The listing builds one solid part. Answer for the finished solid, in the listing's coordinates (mm). A direction names the side the tool comes from. Give positions to 0.01 mm unless a question says otherwise; leave off trailing zeros. Order: outer loops, then holes, each group sorted by start corner. A loop starts at its lowest first (then second) coordinate and runs counter-clockwise, first axis right, second up.
```python
from build123d import *

# Parameters (mm, degrees)
F0_W         = 42
F0_H         = 54
F1_DEPTH     = 8
F2_W         = 39
F2_H         = 50
F3_DEPTH     = 7.2
F5_DEPTH     = 7.2
F6_W         = 20.5
F6_H         = 6.5
F6_W_2       = 18
F6_W_3       = 26.5
F7_DEPTH     = 8.001
F9_DEPTH     = 10
F10_SIZE     = 0.5
F11_T1_DEPTH = 17.5
F12_W        = 39
F12_H        = 3.45
F13_DEPTH    = 7.2
F16_DEPTH    = 1
F19_DEPTH    = 1
F20_SIZE     = 6
F22_W        = 20.5
F22_H        = 6.5
F23_DEPTH    = 0.8


# Not quite as in the source:
# - a fillet or chamfer that OpenCascade refuses, or shapes differently, is made with other operations: its cross-section is extruded or revolved along the edge and cut away or added


with BuildPart() as f1:
    # F0 (on Top) → F1 (new body)
    with BuildSketch(Plane.XY):
        with Locations((0, 27)):
            Rectangle(F0_W, F0_H)
    extrude(amount=F1_DEPTH)

    # F2 (on face) → F3 (cut)
    with BuildSketch(Plane.XY.offset(8)):
        with Locations((0, 27)):
            Rectangle(F2_W, F2_H)
    extrude(amount=-F3_DEPTH, mode=Mode.SUBTRACT)

    # F4 (on face) → F5 (cut, through all)
    with BuildSketch(Plane.XY.offset(8)):
        with BuildLine():
            Line((-19.5, 52), (-17.7, 52))
            ThreePointArc((-17.7, 52), (-19.016227766, 52.9486832981), (-19.5, 51.4))
            Line((-19.5, 51.4), (-19.5, 52))
        make_face()
        with BuildLine():
            ThreePointArc((-19.5, 51.4), (-18.383772234, 51.0513167019), (-17.7, 52))
            Line((-17.7, 52), (-19.5, 52))
            Line((-19.5, 52), (-19.5, 51.4))
        make_face()
        with BuildLine():
            Line((19.5, 52), (17.7, 52))
            ThreePointArc((17.7, 52), (18.383772234, 51.0513167019), (19.5, 51.4))
            Line((19.5, 51.4), (19.5, 52))
        make_face()
        with BuildLine():
            ThreePointArc((19.7, 52), (18.7, 53), (17.7, 52))
            Line((17.7, 52), (19.5, 52))
            Line((19.5, 52), (19.5, 51.4))
            ThreePointArc((19.5, 51.4), (19.6486832981, 51.683772234), (19.7, 52))
        make_face()
        with BuildLine():
            Line((19.5, 2), (19.5, 2.6))
            ThreePointArc((19.5, 2.6), (18.383772234, 2.9486832981), (17.7, 2))
            Line((17.7, 2), (19.5, 2))
        make_face()
        with BuildLine():
            ThreePointArc((-17.7, 2), (-18.383772234, 2.9486832981), (-19.5, 2.6))
            Line((-19.5, 2.6), (-19.5, 2))
            Line((-19.5, 2), (-17.7, 2))
        make_face()
        with BuildLine():
            Line((-19.5, 2), (-19.5, 2.6))
            ThreePointArc((-19.5, 2.6), (-19.016227766, 1.0513167019), (-17.7, 2))
            Line((-17.7, 2), (-19.5, 2))
        make_face()
        with BuildLine():
            ThreePointArc((19.7, 2), (19.6486832981, 2.316227766), (19.5, 2.6))
            Line((19.5, 2.6), (19.5, 2))
            Line((19.5, 2), (17.7, 2))
            ThreePointArc((17.7, 2), (18.7, 1), (19.7, 2))
        make_face()
    extrude(amount=-F5_DEPTH, mode=Mode.SUBTRACT)

    # F6 (on face) → F7 (cut, through all)
    with BuildSketch(Plane.XY.offset(8)):
        with Locations((9.5, 5)):
            Rectangle(F6_W, F6_H)
        with Locations((10.75, 16.1)):
            Rectangle(F6_W_2, F6_H)
        with Locations((-10.75, 16.1)):
            Rectangle(F6_W_2, F6_H)
        with Locations((6.5, 38.3)):
            Rectangle(F6_W_3, F6_H)
    extrude(amount=-F7_DEPTH, mode=Mode.SUBTRACT)

    # F8 (on face) → F9 (join)
    with BuildSketch(Plane.XZ):
        Polygon((-15.25, 2), (-15.25, 8), (-16, 8), (-16, 0), (16, 0), (16, 8), (15.25, 8), (15.25, 2), align=None)
    extrude(amount=F9_DEPTH)

    # F10
    f10_edges = [f1.edges().sort_by_distance(p)[0] for p in [
        (16, -5, 0),
        (18.5, 0, 0),
        (21, 27, 0),
        (-16, -5, 0),
        (-18.5, 0, 0),
        (-21, 27, 0),
        (0, 54, 0),
        (0, -10, 0),
    ]]
    chamfer(f10_edges, length=F10_SIZE)

    # F11: fillet of radius 2 on 4 edges, made by hand

    # F11_s2 → F11_t1 (cut)
    with BuildSketch(Plane.XY.offset(-4.5)):
        with BuildLine():
            ThreePointArc((21, 2), (20.4142135624, 0.5857864376), (19, 0))
            Line((19, 0), (21, 0))
            Line((21, 0), (21, 2))
        make_face()
        with BuildLine():
            ThreePointArc((19, 54), (20.4142135624, 53.4142135624), (21, 52))
            Line((21, 52), (21, 54))
            Line((21, 54), (19, 54))
        make_face()
        with BuildLine():
            ThreePointArc((-21, 2), (-20.4142135624, 0.5857864376), (-19, 0))
            Line((-19, 0), (-21, 0))
            Line((-21, 0), (-21, 2))
        make_face()
        with BuildLine():
            ThreePointArc((-21, 52), (-20.4142135624, 53.4142135624), (-19, 54))
            Line((-19, 54), (-21, 54))
            Line((-21, 54), (-21, 52))
        make_face()
    extrude(amount=F11_T1_DEPTH, mode=Mode.SUBTRACT)

    # F12 (on face) → F13 (join, through all)
    with BuildSketch(Plane.XY.offset(8)):
        with Locations((0, 10.975)):
            Rectangle(F12_W, F12_H)
        with Locations((0, 33.175)):
            Rectangle(F12_W, F12_H)
    extrude(amount=-F13_DEPTH)

    # F15 (on offset) → F16 (join, symmetric)
    with BuildSketch(Plane.YZ.offset(-14.5)):
        Polygon((13.2, 8), (12.7, 8), (12.7, 7.3660254038), (13.2, 7.5), align=None)
        Polygon((52, 7.3660254038), (52, 8), (51.5, 8), (51.5, 7.5), align=None)
    extrude(amount=F16_DEPTH, both=True)

    # F18 (on offset) → F19 (join, symmetric)
    with BuildSketch(Plane.YZ.offset(14.5)):
        Polygon((13.2, 7.5), (13.2, 8), (12.7, 8), (12.7, 7.3660254038), align=None)
        Polygon((51.5, 7.5), (52, 7.3660254038), (52, 8), (51.5, 8), align=None)
    extrude(amount=F19_DEPTH, both=True)

    # F20
    f20_edges = [f1.edges().sort_by_distance(p)[0] for p in [
        (-15.625, -10, 8),
        (15.625, -10, 8),
    ]]
    chamfer(f20_edges, length=F20_SIZE)

    # F22 (on face) → F23 (join)
    with BuildSketch(Plane(origin=(0, 0, 0), x_dir=(1, 0, 0), z_dir=(0, 0, -1))):
        with Locations((9.5, -5)):
            Rectangle(F22_W, F22_H)
    extrude(amount=-F23_DEPTH)


solid = f1.part
```
1) A tool of negligible diameter and unlimited length cuts with its end or side. For faces 3 (the flat face through (17, 0, 4)), 4 (the flat face through (-19.5, 43, 4)), 5 (the flat face through (-15.25, -4, 4)), from which of +Z, -Z, +X, -X, +Y, -Y can it reach the whole face along a straight path? Write none if from no direction.
Geometry says:
face 3: +Z, -Z, +X, -Y
face 4: +Z
face 5: +Z, -Y
2) Find section C-C (y = -2). Write down the section's boundary in (x, z), then the cut area to 4 significant figures.
Geometry says:
outline: (-16, 0.5) - (-15.5, 0) - (15.5, 0) - (16, 0.5) - (16, 8) - (15.25, 8) - (15.25, 2) - (-15.25, 2) - (-15.25, 8) - (-16, 8) - close
area: 72.75 mm2
3) Straight lines are drawn through the part: probe 1 along Y at (x, z) = (-4.5, 6.5); probe 2 along Y at (x, z) = (-18.7, 3.75); probe 3 along X at (y, z) = (5, 6). For each, find the intervals that lie inside material, in ascending order.
Geometry says:
probe 1: y = 0 to 2, 9.25 to 12.7, 31.45 to 34.9, 52 to 54
probe 2: y = 0 to 1, 9.25 to 12.7, 31.45 to 34.9, 53 to 54
probe 3: x = -21 to -19.5, 19.75 to 21
4) For a pull along X with two mould halves and no side action, classify faces 1 (the flat face through (19.5, 46, 4)), 2 (the flat face through (-18, 0, 4)) as +X half, -X half, draft (parallel to the pull), parting line (faces both ways), or undercut.
Geometry says:
face 1: undercut
face 2: draft
5) Given P1, Ø1.8, axis at y = -3.5, z = 4, coming from the -X side; P2, Ø5, axis at x = 15, y = 21.5, coming from the +Z side, each flat-ended and moving along its own axis, determine where each tip first touches the part or whether it passes through.
Geometry says:
P1: stops at x = -16
P2: stops at z = 0.8
6) Find section A-A (x = -3). Write down the section's boundary in (y, z), then the cut area to 3 significant figures.
Geometry says:
outline: (-10, 0.5) - (-9.5, 0) - (12.85, 0) - (12.85, 0.8) - (12.7, 0.8) - (12.7, 8) - (9.25, 8) - (9.25, 0.8) - (2, 0.8) - (2, 8) - (0, 8) - (0, 2) - (-10, 2) - close; (19.35, 0) - (35.05, 0) - (35.05, 0.8) - (34.9, 0.8) - (34.9, 8) - (31.45, 8) - (31.45, 0.8) - (19.35, 0.8) - close; (41.55, 0) - (53.5, 0) - (54, 0.5) - (54, 8) - (52, 8) - (52, 0.8) - (41.55, 0.8) - close
area: 131 mm2
7) Find section B-B (x = -17). Write down the section's boundary in (y, z), then the cut area to 3 significant figures.
Geometry says:
outline: (0, 0.5) - (0.5, 0) - (12.85, 0) - (12.85, 0.8) - (12.7, 0.8) - (12.7, 8) - (9.25, 8) - (9.25, 0.8) - (2, 0.8) - (2, 8) - (0, 8) - close; (19.35, 0) - (53.5, 0) - (54, 0.5) - (54, 8) - (52, 8) - (52, 0.8) - (34.9, 0.8) - (34.9, 8) - (31.45, 8) - (31.45, 0.8) - (19.35, 0.8) - close
area: 116 mm2
8) Find section D-D (z = 4.5). Count the separate pieces of the cut face and the enclosed holes in it, then the cut area to 3 significant figures.
Geometry says:
separate pieces: 1
enclosed holes: 3
area: 577 mm2
